Autodesk Inventor part; units mm, degrees
ref_plane "YZ Plane" through (0, 0, 0) normal (1, 0, 0) x (0, 1, 0)
ref_plane "XZ Plane" through (0, 0, 0) normal (0, 1, 0) x (-1, 0, 0)
ref_plane "XY Plane" through (0, 0, 0) normal (0, 0, 1) x (1, 0, 0)
sketch "Sketch2" plane through (0, 0, 0) normal (0, 1, 0) x (-1, 0, 0)
  line L0 (0, 0) -> (20, 0)
  line L1 (20, 0) -> (20, -20)
  line L2 (20, -20) -> (0, -20)
  line L3 (0, -20) -> (0, 0)
  line L4 (20, 0) -> (0, -20) construction
  line L5 (20, -20) -> (0, 0) construction
  circle A0 centre (15.6569, -4.3431) radius 1.5
  circle A1 centre (16.7175, -16.7175) radius 1.5
  circle A2 centre (3.2825, -3.2825) radius 1.5
  circle A3 centre (4.3431, -15.6569) radius 1.5
  circle A4 centre (10, -10) radius 4.5
  line L6 (20, -20) -> (25, -20)
  line L7 (25, -20) -> (25, 0)
  line L8 (25, 0) -> (20, 0)
  line L9 (20, 0) -> (20, -20)
  line L10 (0, -20) -> (-5, -20)
  line L11 (-5, -20) -> (-5, 0)
  line L12 (-5, 0) -> (0, 0)
  line L13 (0, 0) -> (0, -20)
  arc A5 (25, -20) -> (25, 0) centre (25, -10) ccw
  arc A6 (-5, 0) -> (-5, -20) centre (-5, -10) ccw
  circle A7 centre (31, -10) radius 1.5
  circle A8 centre (-11, -10) radius 1.5
  dimension "d37" = 3
  dimension "d38" = 3
  dimension "d39" = 3
  dimension "d40" = 3
  dimension "d41" = 9.5
  dimension "d42" = 9.5
  dimension "d43" = 8
  dimension "d44" = 8
  dimension "d60" = 20
  dimension "d61" = 9
  dimension "d66" = 5
  dimension "d67" = 5
  dimension "d68" = 3
  dimension "d69" = 3
  dimension "d70" = 6
  dimension "d71" = 6
extrude "Extrusion2" add sketch "Sketch2" along normal blind 2
sketch "Sketch3" plane through (0, 2, 0) normal (0, 1, 0) x (1, 0, 0)
  line L0 (5, 20) -> (-25, 20)
  arc A0 (-25, 20) -> (-25, 0) centre (-25, 10) ccw
  line L1 (-25, 0) -> (5, 0)
  arc A1 (5, 0) -> (5, 20) centre (5, 10) ccw
  circle A2 centre (-16.7175, 16.7175) radius 1.5
  circle A3 centre (-3.2825, 3.2825) radius 1.5
  circle A4 centre (-10, 10) radius 4.5
  circle A5 centre (-4.3431, 15.6569) radius 1.5
  circle A6 centre (-15.6569, 4.3431) radius 1.5
  circle A7 centre (-31, 10) radius 1.5
  circle A8 centre (11, 10) radius 1.5
  point P0 (0, 0)
properties part number "Motor_mount_plate"
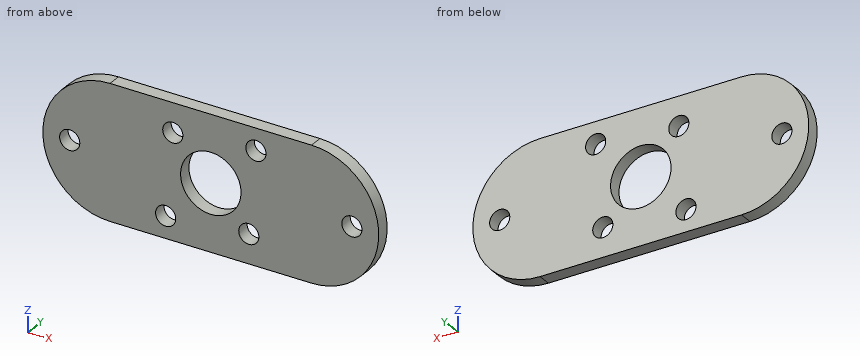
Geometry: final body of the model. Coordinates: model frame, mm. Round coordinates to 2 decimals unless told otherwise and drop trailing zeros. Write each loop counter-clockwise with the first axis right and the second up, starting at its lowest first coordinate (ties: lowest second). Pieces come first, ordered by that corner, then holes. Notation, with made-up numbers: M -15.75,13 L 30.25,13 A6 ccw 30.25,20 Z; hole C 29.25,59 d8. An arc over 180 degrees is marked long. Write item = value, one per line.
Item 1: Section query C-C on y = 0.4. Return loops of the section in (x, z).
Findings:
outline = M -25,-20 L 5,-20 A10 ccw 5,0 L -25,0 A10 ccw Z; hole C -31,-10 d3; hole C -16.72,-16.72 d3; hole C -15.66,-4.34 d3; hole C -10,-10 d9; hole C -4.34,-15.66 d3; hole C -3.28,-3.28 d3; hole C 11,-10 d3
Item 2: Section query A-A on x = -31. Return loops of the section in (y, z), then the cut area to 3 significant figures.
Findings:
outline = M 0,-18 L 2,-18 L 2,-11.5 L 0,-11.5 Z; M 0,-8.5 L 2,-8.5 L 2,-2 L 0,-2 Z
area = 26.0 mm^2
Item 3: Material intervals for line 1 along X through (y, z) = (0.2, -15.5); line 2 along X through (y, z) = (0.55, -3.5); line 3 along X through (y, z) = (0.3, -12.5), sorted ascending. Write a range as [from, to].
Findings:
line_1 = [-33.35, -17.59], [-15.84, -5.83], [-2.85, 13.35]
line_2 = [-32.6, -16.9], [-14.42, -4.77], [-1.8, 12.6]
line_3 = [-34.68, -13.74], [-6.26, 14.68]
Item 4: Section query D-D on z = -13.5. Return loops of the section in (x, y), then the cut area to 3 significant figures.
Findings:
outline = M -34.37,0 L -12.83,0 L -12.83,2 L -34.37,2 Z; M -7.17,0 L 14.37,0 L 14.37,2 L -7.17,2 Z
area = 86.2 mm^2
Item 5: Section query B-B on z = -10. Return loops of the section in (x, y).
Findings:
outline = M -35,0 L -32.5,0 L -32.5,2 L -35,2 Z; M -29.5,0 L -14.5,0 L -14.5,2 L -29.5,2 Z; M -5.5,0 L 9.5,0 L 9.5,2 L -5.5,2 Z; M 12.5,0 L 15,0 L 15,2 L 12.5,2 Z
